from build123d import *

# Parameters (mm, degrees)
F1_DEPTH = 15
F2_T     = -2.5
F3_DEPTH = 3
F4_DEPTH = 4
F5_R     = 0.5
F6_R     = 1
F7_START = 12.5
F0_R     = 1
F7_DEPTH = 2.5


with BuildPart() as f1:
    # F0 (on Top) → F1 (new body)
    with BuildSketch(Plane.XY):
        with BuildLine():
            ThreePointArc((75, 7.5), (73.5355339059, 11.0355339059), (70, 12.5))
            Line((70, 12.5), (61.1287162602, 12.5))
            Line((61.1287162602, 12.5), (41.6287162602, 12.5))
            Line((41.6287162602, 12.5), (-41.6287162602, 12.5))
            Line((-41.6287162602, 12.5), (-61.1287162602, 12.5))
            Line((-61.1287162602, 12.5), (-70, 12.5))
            ThreePointArc((-70, 12.5), (-73.5355339059, 11.0355339059), (-75, 7.5))
            Line((-75, 7.5), (-75, -7.5))
            ThreePointArc((-75, -7.5), (-73.5355339059, -11.0355339059), (-70, -12.5))
            Line((-70, -12.5), (70, -12.5))
            ThreePointArc((70, -12.5), (73.5355339059, -11.0355339059), (75, -7.5))
            Line((75, -7.5), (75, 7.5))
        make_face()
        with BuildLine():
            Line((-66.8997643389, 3), (66.8997643389, 3))
            ThreePointArc((66.8997643389, 3), (68.0313018263, 2.5313018263), (68.5, 1.3997643389))
            Line((68.5, 1.3997643389), (68.5, -1.3997643389))
            ThreePointArc((68.5, -1.3997643389), (68.0313018263, -2.5313018263), (66.8997643389, -3))
            Line((66.8997643389, -3), (-66.8997643389, -3))
            ThreePointArc((-66.8997643389, -3), (-68.0313018263, -2.5313018263), (-68.5, -1.3997643389))
            Line((-68.5, -1.3997643389), (-68.5, 1.3997643389))
            ThreePointArc((-68.5, 1.3997643389), (-68.0313018263, 2.5313018263), (-66.8997643389, 3))
        make_face(mode=Mode.SUBTRACT)
        with BuildLine():
            ThreePointArc((68.5, 1.3997643389), (68.0313018263, 2.5313018263), (66.8997643389, 3))
            Line((66.8997643389, 3), (-66.8997643389, 3))
            ThreePointArc((-66.8997643389, 3), (-68.0313018263, 2.5313018263), (-68.5, 1.3997643389))
            Line((-68.5, 1.3997643389), (-68.5, -1.3997643389))
            ThreePointArc((-68.5, -1.3997643389), (-68.0313018263, -2.5313018263), (-66.8997643389, -3))
            Line((-66.8997643389, -3), (66.8997643389, -3))
            ThreePointArc((66.8997643389, -3), (68.0313018263, -2.5313018263), (68.5, -1.3997643389))
            Line((68.5, -1.3997643389), (68.5, 1.3997643389))
        make_face()
        with BuildLine():
            ThreePointArc((67.5, -0.3997643389), (67.0313018263, -1.5313018263), (65.8997643389, -2))
            Line((65.8997643389, -2), (-65.8997643389, -2))
            ThreePointArc((-65.8997643389, -2), (-67.0313018263, -1.5313018263), (-67.5, -0.3997643389))
            Line((-67.5, -0.3997643389), (-67.5, 0.3997643389))
            ThreePointArc((-67.5, 0.3997643389), (-67.0313018263, 1.5313018263), (-65.8997643389, 2))
            Line((-65.8997643389, 2), (65.8997643389, 2))
            ThreePointArc((65.8997643389, 2), (67.0313018263, 1.5313018263), (67.5, 0.3997643389))
            Line((67.5, 0.3997643389), (67.5, -0.3997643389))
        make_face(mode=Mode.SUBTRACT)
        with BuildLine():
            Line((-65.8997643389, -2), (65.8997643389, -2))
            ThreePointArc((65.8997643389, -2), (67.0313018263, -1.5313018263), (67.5, -0.3997643389))
            Line((67.5, -0.3997643389), (67.5, 0.3997643389))
            ThreePointArc((67.5, 0.3997643389), (67.0313018263, 1.5313018263), (65.8997643389, 2))
            Line((65.8997643389, 2), (-65.8997643389, 2))
            ThreePointArc((-65.8997643389, 2), (-67.0313018263, 1.5313018263), (-67.5, 0.3997643389))
            Line((-67.5, 0.3997643389), (-67.5, -0.3997643389))
            ThreePointArc((-67.5, -0.3997643389), (-67.0313018263, -1.5313018263), (-65.8997643389, -2))
        make_face()
    extrude(amount=F1_DEPTH)

    # F2
    f2_openings = [f1.faces().sort_by_distance(p)[0] for p in [
        (0, 0, 15),
    ]]
    offset(amount=F2_T, openings=f2_openings)

    # F0 (on Top) → F3 (cut)
    with BuildSketch(Plane.XY):
        with BuildLine():
            Line((-65.8997643389, -2), (65.8997643389, -2))
            ThreePointArc((65.8997643389, -2), (67.0313018263, -1.5313018263), (67.5, -0.3997643389))
            Line((67.5, -0.3997643389), (67.5, 0.3997643389))
            ThreePointArc((67.5, 0.3997643389), (67.0313018263, 1.5313018263), (65.8997643389, 2))
            Line((65.8997643389, 2), (-65.8997643389, 2))
            ThreePointArc((-65.8997643389, 2), (-67.0313018263, 1.5313018263), (-67.5, 0.3997643389))
            Line((-67.5, 0.3997643389), (-67.5, -0.3997643389))
            ThreePointArc((-67.5, -0.3997643389), (-67.0313018263, -1.5313018263), (-65.8997643389, -2))
        make_face()
    extrude(amount=F3_DEPTH, mode=Mode.SUBTRACT)

    # F0 (on Top) → F4 (join)
    with BuildSketch(Plane.XY):
        with BuildLine():
            ThreePointArc((68.5, 1.3997643389), (68.0313018263, 2.5313018263), (66.8997643389, 3))
            Line((66.8997643389, 3), (-66.8997643389, 3))
            ThreePointArc((-66.8997643389, 3), (-68.0313018263, 2.5313018263), (-68.5, 1.3997643389))
            Line((-68.5, 1.3997643389), (-68.5, -1.3997643389))
            ThreePointArc((-68.5, -1.3997643389), (-68.0313018263, -2.5313018263), (-66.8997643389, -3))
            Line((-66.8997643389, -3), (66.8997643389, -3))
            ThreePointArc((66.8997643389, -3), (68.0313018263, -2.5313018263), (68.5, -1.3997643389))
            Line((68.5, -1.3997643389), (68.5, 1.3997643389))
        make_face()
        with BuildLine():
            ThreePointArc((67.5, -0.3997643389), (67.0313018263, -1.5313018263), (65.8997643389, -2))
            Line((65.8997643389, -2), (-65.8997643389, -2))
            ThreePointArc((-65.8997643389, -2), (-67.0313018263, -1.5313018263), (-67.5, -0.3997643389))
            Line((-67.5, -0.3997643389), (-67.5, 0.3997643389))
            ThreePointArc((-67.5, 0.3997643389), (-67.0313018263, 1.5313018263), (-65.8997643389, 2))
            Line((-65.8997643389, 2), (65.8997643389, 2))
            ThreePointArc((65.8997643389, 2), (67.0313018263, 1.5313018263), (67.5, 0.3997643389))
            Line((67.5, 0.3997643389), (67.5, -0.3997643389))
        make_face(mode=Mode.SUBTRACT)
    extrude(amount=-F4_DEPTH)

    # F5
    f5_edges = [f1.edges().sort_by_distance(p)[0] for p in [
        (0, -2, -4),
        (-67.031302, -1.531302, -4),
    ]]
    fillet(f5_edges, radius=F5_R)

    # F6
    f6_edges = [f1.edges().sort_by_distance(p)[0] for p in [
        (0, 2, 2.5),
    ]]
    fillet(f6_edges, radius=F6_R)

    # F0 (on Top) → F7 (join)
    with BuildSketch(Plane.XY.offset(F7_START)):
        with BuildLine():
            Line((41.6287162602, 12.5), (61.1287162602, 12.5))
            ThreePointArc((61.1287162602, 12.5), (58.3002891354, 13.6715728753), (57.1287162602, 16.5))
            Line((57.1287162602, 16.5), (57.1287162602, 88.5))
            ThreePointArc((57.1287162602, 88.5), (55.9571433849, 91.3284271247), (53.1287162602, 92.5))
            Line((53.1287162602, 92.5), (49.6287162602, 92.5))
            ThreePointArc((49.6287162602, 92.5), (46.8002891354, 91.3284271247), (45.6287162602, 88.5))
            Line((45.6287162602, 88.5), (45.6287162602, 16.5))
            ThreePointArc((45.6287162602, 16.5), (44.4571433849, 13.6715728753), (41.6287162602, 12.5))
        make_face()
        with Locations((51.3787162602, 22.5)):
            Circle(F0_R, mode=Mode.SUBTRACT)
        with BuildLine():
            Line((-61.1287162602, 12.5), (-41.6287162602, 12.5))
            ThreePointArc((-41.6287162602, 12.5), (-44.4571433849, 13.6715728753), (-45.6287162602, 16.5))
            Line((-45.6287162602, 16.5), (-45.6287162602, 88.5))
            ThreePointArc((-45.6287162602, 88.5), (-46.8002891354, 91.3284271247), (-49.6287162602, 92.5))
            Line((-49.6287162602, 92.5), (-53.1287162602, 92.5))
            ThreePointArc((-53.1287162602, 92.5), (-55.9571433849, 91.3284271247), (-57.1287162602, 88.5))
            Line((-57.1287162602, 88.5), (-57.1287162602, 16.5))
            ThreePointArc((-57.1287162602, 16.5), (-58.3002891354, 13.6715728753), (-61.1287162602, 12.5))
        make_face()
        with Locations((-51.3787162602, 22.5)):
            Circle(F0_R, mode=Mode.SUBTRACT)
    extrude(amount=F7_DEPTH)


solid = f1.part
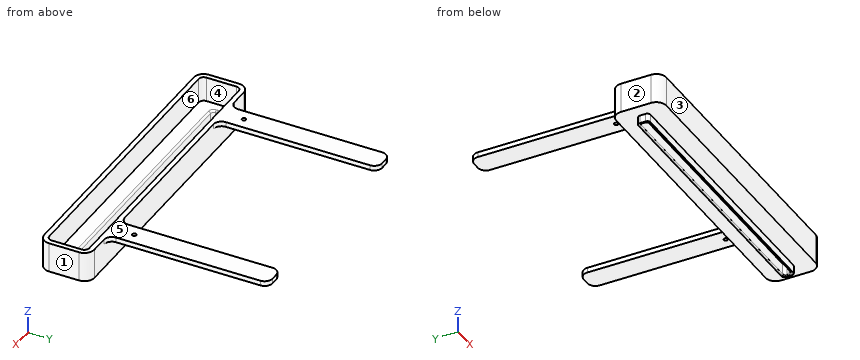
Design review of the part built by this model. Coordinates are the model's own, in mm. Face numbers are marked on the shaded views. A direction names the side the tool comes from. Give positions to 0.01 mm unless a question says otherwise; leave off trailing zeros. Order: outer loops, then holes, each group sorted by start corner. A loop starts at its lowest first (then second) coordinate and runs counter-clockwise, first axis right, second up. Notation, with made-up numbers: (44.5, -36) - (64.5, -36) arc R38 cw to (64.5, 3) - close; hole circle Ø6 at (20.25, 24). An arc over 180 degrees is marked (long way). Write item = value, one per line. Start each with the question number.
Q1. We need section A-A on z = 11. State the section outline as (x, y) points, plus the area to 3 significant figures.
Q2. We need section D-D on y = 14. State the section outline as (x, z) points, plus the area to 3 significant figures.
Q3. We need section C-C on y = 46.5. State the section outline as (x, z) points.
Q4. To check wall thickness, follow L1, parallel to Y at x = 21, z = 4; L2, parallel to Y at x = 20, z = -2; L3, parallel to Z at x = 59, y = 4.5. State the ranges of each line that lie inside material, in increasing order. Write a range as from..to.
Q5. Tool access review of the marked faces 5 and 6: name each direction out of +Z, -Z, +X, -X, +Y, -Y from which nothing blocks a thin tool from reaching the whole face with its end or side.
Q6. Mouldability with a two-part tool opening along X and no side actions: class the marked faces 1, 2, 3 and 4 as released by +X, released by -X, zero draft, split by the parting line, or undercut.
Q7. We need section B-B on x = 30.5. State the section outline as (y, z) points.
Q8. Clearance check with flat-ended pins moving along their axes: pin 1 Ø0.8 at (y, z) = (0, -2) entering from -X; pin 2 Ø3 at (y, z) = (53.5, 13.5) entering from +X; pin 3 Ø2 at (y, z) = (60.5, 14) entering from -X; pin 4 Ø1.6 at (x, y) = (-51.38, 22.5) entering from -Z. State where each tip first meets the part, or that it passes through.
Working result:
q1.outline = (-75, -7.5) arc R5 ccw to (-70, -12.5) - (70, -12.5) arc R5 ccw to (75, -7.5) - (75, 7.5) arc R5 ccw to (70, 12.5) - (-70, 12.5) arc R5 ccw to (-75, 7.5) - close; hole (-72.5, -7.5) arc R2.5 ccw to (-70, -10) - (70, -10) arc R2.5 ccw to (72.5, -7.5) - (72.5, 7.5) arc R2.5 ccw to (70, 10) - (-70, 10) arc R2.5 ccw to (-72.5, 7.5) - close
q1.area = 834 mm²
q2.outline = (-58.01, 12.5) - (-44.75, 12.5) - (-44.75, 15) - (-58.01, 15) - close; (44.75, 12.5) - (58.01, 12.5) - (58.01, 15) - (44.75, 15) - close
q2.area = 66.3 mm²
q3.outline = (-57.13, 12.5) - (-45.63, 12.5) - (-45.63, 15) - (-57.13, 15) - close; (45.63, 12.5) - (57.13, 12.5) - (57.13, 15) - (45.63, 15) - close
q4.L1 = -12.5..-10, 10..12.5
q4.L2 = -3..-2, 2..3
q4.L3 = 0..2.5
q5.face_5 = +Z, +X, -X, +Y, -Y
q5.face_6 = +Z
q6.face_1 = released by +X
q6.face_2 = released by -X
q6.face_3 = zero draft
q6.face_4 = undercut
q7.outline = (-12.5, 0) - (-3, 0) - (-3, -4) - (-2.5, -4) arc R0.5 ccw to (-2, -3.5) - (-2, 1.5) arc R1 ccw to (-3, 2.5) - (-10, 2.5) - (-10, 15) - (-12.5, 15) - close; (2, -3.5) arc R0.5 ccw to (2.5, -4) - (3, -4) - (3, 0) - (12.5, 0) - (12.5, 15) - (10, 15) - (10, 2.5) - (3, 2.5) arc R1 ccw to (2, 1.5) - close
q8.pin_1 = -68.5
q8.pin_2 = 57.13
q8.pin_3 = -57.13
q8.pin_4 = through
